from build123d import *

# Parameters (mm, degrees)
SKETCH1_W           = 38
SKETCH1_H           = 13
SKETCH1_R           = 1.6
BOSS_EXTRUDE1_DEPTH = 3.6
SKETCH2_W           = 24
SKETCH2_H           = 1.4
CUT_EXTRUDE1_DEPTH  = 24.301502098
CHAMFER1_SIZE       = 1.5
CHAMFER1_SIZE2      = 1.350606066


with BuildPart() as part:
    # Sketch1 → Boss-Extrude1 (new body)
    with BuildSketch(Plane.XY):
        Rectangle(SKETCH1_W, SKETCH1_H)
        with Locations((-15, 2)):
            Circle(SKETCH1_R, mode=Mode.SUBTRACT)
        with Locations(Location((15, 2, 0), (0, 0, 180))):
            Circle(SKETCH1_R, mode=Mode.SUBTRACT)
    extrude(amount=BOSS_EXTRUDE1_DEPTH)

    # Sketch2 → Cut-Extrude1 (cut, through all)
    with BuildSketch(Plane(origin=(0, 6.5, 0), x_dir=(1, 0, 0), z_dir=(0, 1, 0))):
        with Locations((0, -0.7)):
            Rectangle(SKETCH2_W, SKETCH2_H)
    extrude(amount=-CUT_EXTRUDE1_DEPTH, mode=Mode.SUBTRACT)

    # Chamfer1
    chamfer1_edges = [part.edges().sort_by_distance(p)[0] for p in [
        (-16.6, 2, 3.6),
        (16.6, 2, 3.6),
    ]]
    chamfer1_side = [part.faces().sort_by_distance(p)[0] for p in [
        (0, -0.067313028, 3.6),
    ]]
    chamfer(chamfer1_edges, length=CHAMFER1_SIZE, length2=CHAMFER1_SIZE2, reference=chamfer1_side[0])


solid = part.part
Check sheet for the modelled part. Datum: model origin and axes. Units: mm. A direction names the side the tool comes from. Coordinates: 2 decimals unless noted, no trailing zeros. Loops run counter-clockwise (first coordinate to the right, second up) from the corner with the lowest first, then second, coordinate; pieces in that order, holes last. Notation, with made-up numbers: (89.25, 26) -> (141.25, 26) arc R22 cw to (141.25, 48) -> close; hole circle Ø3 at (-25.5, -22). An arc over 180 degrees is marked (long way). Write item = value, one per line. Start each with the question number.
1. Section check A-A on y = 2. Record the cut outline in (x, z).
2. Draft check along X on faces 1 (the flat face through (0, 0, 3.6)), 2 (the flat face through (-19, 0, 2)), 3 (the cylindrical face through (-16.6, 2.07, 1.11)), 4 (the flat face through (-12, 0, 1)). Enter one of: released by +X, released by -X, zero draft, split by the parting line, or undercut.
3. Material ranges on line 1 (X direction, y = -4, z = 1); line 2 (X direction, y = 3.25, z = 0.3); line 3 (X direction, y = 0.75, z = 3.55), recorded low to high.
4. Tool access check on faces 5 (the flat face through (12, 0, 1)), 6 (the flat face through (-16, 0, 0)). Record the directions out of +Z, -Z, +X, -X, +Y, -Y that give a thin tool (end or side, any length) a straight path to the whole face; none if there is none.
5. Depth check by flat-ended pin: P1, Ø6, axis at x = 5, y = 4, coming from the -Z side; P2, Ø4, axis at x = 15, y = 2, coming from the +Z side. Enter the tip coordinate at first touch or a pass-through.
6. Section check B-B on z = 0.35. Record the cut outline in (x, y).
7. Section check C-C on x = -15. Record the cut outline in (y, z).
8. Section check D-D on z = 2.95. Record the cut outline in (x, y).
Responses:
q1.outline = (-19, 0) -> (-16.6, 0) -> (-16.6, 2.25) -> (-18.1, 3.6) -> (-19, 3.6) -> close; (-13.4, 0) -> (-12, 0) -> (-12, 1.4) -> (12, 1.4) -> (12, 0) -> (13.4, 0) -> (13.4, 2.25) -> (11.9, 3.6) -> (-11.9, 3.6) -> (-13.4, 2.25) -> close; (16.6, 0) -> (19, 0) -> (19, 3.6) -> (18.1, 3.6) -> (16.6, 2.25) -> close
q2.face_1 = zero draft
q2.face_2 = released by -X
q2.face_3 = undercut
q2.face_4 = undercut
q3.line_1 = -19 to -12, 12 to 19
q3.line_2 = -19 to -16, -14 to -12, 12 to 14, 16 to 19
q3.line_3 = -19 to -17.78, -12.22 to 12.22, 17.78 to 19
q4.face_5 = -Z, +Y, -Y
q4.face_6 = -Z, +X, -X, +Y, -Y
q5.P1 = 1.4
q5.P2 = 2.61
q6.outline = (-19, -6.5) -> (-12, -6.5) -> (-12, 6.5) -> (-19, 6.5) -> close; (12, -6.5) -> (19, -6.5) -> (19, 6.5) -> (12, 6.5) -> close; hole circle Ø3.2 at (-15, 2); hole circle Ø3.2 at (15, 2)
q7.outline = (-6.5, 0) -> (0.4, 0) -> (0.4, 2.25) -> (-1.1, 3.6) -> (-6.5, 3.6) -> close; (3.6, 0) -> (6.5, 0) -> (6.5, 3.6) -> (5.1, 3.6) -> (3.6, 2.25) -> close
q8.outline = (-19, -6.5) -> (19, -6.5) -> (19, 6.5) -> (-19, 6.5) -> close; hole circle Ø4.76 at (-15, 2); hole circle Ø4.76 at (15, 2)
